from build123d import *

# Parameters (mm, degrees)
SKETCH1_R                  = 35
SKETCH1_R_2                = 6
SKETCH1_R_3                = 5
SKETCH1_W                  = 50
SKETCH1_H                  = 25
BOSS_EXTRUDE1_DEPTH        = 2.38125
FILLET1_R                  = 4
FILLET2_R                  = 4
FILLET3_R                  = 1
F_4_7_4_7_DIAMETER_HOLE1_D = 4.7


with BuildPart() as part:
    # Sketch1 → Boss-Extrude1 (new body)
    with BuildSketch(Plane(origin=(0, 0, 0), x_dir=(1, 0, 0), z_dir=(0, 1, 0))):
        with Locations((32.785, 18.724314586)):
            Circle(SKETCH1_R)
        with Locations((32.785, 18.724314586)):
            Circle(SKETCH1_R_2, mode=Mode.SUBTRACT)
        with Locations((65.57, 0)):
            Circle(SKETCH1_R_3)
        Circle(SKETCH1_R_3)
        with Locations((32.785, 65.782929207)):
            Circle(SKETCH1_R_3)
        with Locations((32.785, 53.282929207)):
            Rectangle(SKETCH1_W, SKETCH1_H)
    extrude(amount=BOSS_EXTRUDE1_DEPTH)

    # Fillet1
    fillet1_edges = [part.edges().sort_by_distance(p)[0] for p in [
        (64.966328407, 1.190625, -4.963424282),
        (60.988257258, 1.190625, 2.001907453),
    ]]
    fillet(fillet1_edges, radius=FILLET1_R)

    # Fillet2
    fillet2_edges = [part.edges().sort_by_distance(p)[0] for p in [
        (0.603671593, 1.190625, -4.963424282),
        (4.581742742, 1.190625, 2.001907453),
    ]]
    fillet(fillet2_edges, radius=FILLET2_R)

    # Fillet3
    fillet3_edges = [part.edges().sort_by_distance(p)[0] for p in [
        (37.785, 1.190625, -65.782929207),
        (27.785, 1.190625, -65.782929207),
    ]]
    fillet(fillet3_edges, radius=FILLET3_R)

    # Ø4.7 (4.7) Diameter Hole1 (through all)
    with Locations(Plane(origin=(0, 2.38125, 0), x_dir=(1, 0, 0), z_dir=(0, 1, 0))):
        with Locations((32.785, 65.782929207), (0, 0), (65.57, 0)):
            Hole(F_4_7_4_7_DIAMETER_HOLE1_D / 2)


solid = part.part
Verification items for the finished model (mm, model axes). A direction names the side the tool comes from. Give positions to 0.01 mm unless a question says otherwise; leave off trailing zeros. Write each loop counter-clockwise with the first axis right and the second up, starting at its lowest first coordinate (ties: lowest second). Pieces come first, ordered by that corner, then holes. Notation, with made-up numbers: M -11.5,-26 L 23.5,-26 A26 ccw 23.5,0 Z; hole C 46,16 d3. An arc over 180 degrees is marked long. Put each result on its own line as item: value. Start each with the question number.
1. Draft check along Z on faces 1 (the face through (17, 1, -65.783)), 2 (the face through (0.509, 1.174, 2.294)), 3 (the face through (32, 2.381, -28)), 4 (the face through (-4.395, 1.174, 2.385)). Enter one of: +Z half, -Z half, draft (parallel to the pull), parting line (faces both ways), or undercut.
2. Section check B-B (z = -16). Record the cut outline in (x, y).
3. Go/stop test with flat-tipped pins: pin 1 Ø1 at (y, z) = (1.5, -18.5) entering from -X (3 decimals); pin 2 Ø0.7 at (x, y) = (45, 1.5) entering from -Z; pin 3 Ø7.5 at (x, z) = (0, 0) entering from +Y; pin 4 Ø1.2 at (y, z) = (0.5, -55.5) entering from -X (3 decimals). Record where each tip stops, or that it passes through.
4. Scan lines: line 1 along Z through (x, y) = (32.5, 0.8); line 2 along X through (y, z) = (0.95, -57) (3 decimals); line 3 along Z through (x, y) = (30, 0.4). Record each from-to range of solid material in increasing order. Write a range as [from, to].
5. Section check D-D (y = 1.95). Give the number of separate pieces and of enclosed holes in the cut face, and give its area (3 significant figures).
6. Section check C-C (x = 65). Record the cut outline in (y, z), and give its area (3 significant figures).
7. Set-up check for faces 5 (the face through (7.785, 1, -54)), 6 (the face through (32.384, 1.174, 16.273)), 7 (the face through (57.785, 1, -54)): record each of +Z, -Z, +X, -X, +Y, -Y from which the full face is reachable in a straight line by a thin tool's end or side.
8. Section check A-A (z = 0). Record the cut outline in (x, y).
Answer list:
1. face 1: -Z half
1. face 2: undercut
1. face 3: draft
1. face 4: parting line
2. outline: M -2.11,0 L 27.44,0 L 27.44,2.38 L -2.11,2.38 Z; M 38.13,0 L 67.68,0 L 67.68,2.38 L 38.13,2.38 Z
3. pin 1: x = -2.215
3. pin 2: z = -65.78
3. pin 3: y = 2.38
3. pin 4: x = 7.785
4. line 1: [-70.77, -68.12], [-63.45, -24.72], [-12.73, 16.27]
4. line 2: [7.785, 57.785]
4. line 3: [-69.94, -24.04], [-13.41, 16.16]
5. separate pieces: 1
5. enclosed holes: 4
5. area: 4,630 mm2
6. outline: M 0,-32.41 L 2.38,-32.41 L 2.38,-2.28 L 0,-2.28 Z; M 0,2.28 L 2.38,2.28 L 2.38,4.97 L 0,4.97 Z
6. area: 78.1 mm2
7. face 5: -Z, -X, +Y, -Y
7. face 6: +Z, +Y, -Y
7. face 7: -Z, +X, +Y, -Y
8. outline: M -5,0 L -2.35,0 L -2.35,2.38 L -5,2.38 Z; M 2.35,0 L 63.22,0 L 63.22,2.38 L 2.35,2.38 Z; M 67.92,0 L 70.57,0 L 70.57,2.38 L 67.92,2.38 Z
